from build123d import *

# Parameters (mm, degrees)
F1_DEPTH = 304.8


with BuildPart() as f1:
    # F0 (on Front) → F1 (new body)
    with BuildSketch(Plane.XZ):
        with BuildLine():
            Line((-9.986188, 0), (0, 0))
            Line((0, 0), (109.393812, 0))
            ThreePointArc((109.393812, 0), (110.663812, 0.340295), (111.593517, 1.27))
            Line((111.593517, 1.27), (-8.716188, 1.27))
            ThreePointArc((-8.716188, 1.27), (-10.512239, 2.013949), (-11.256188, 3.81))
            Line((-11.256188, 3.81), (-11.256188, 26.67))
            Line((-11.256188, 26.67), (-12.526188, 26.67))
            Line((-12.526188, 26.67), (-12.526188, 2.54))
            ThreePointArc((-12.526188, 2.54), (-11.782239, 0.743949), (-9.986188, 0))
        make_face()
    extrude(amount=-F1_DEPTH)


solid = f1.part
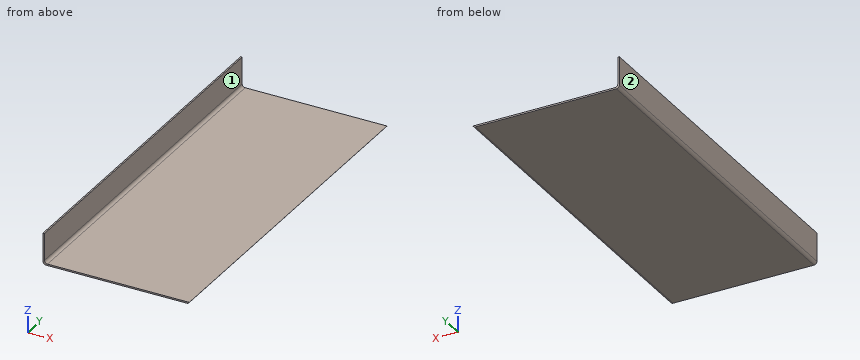
Could you check a few things on this model? Use its own coordinates, in mm. Face numbers are marked on the shaded views. A direction names the side the tool comes from. Give positions to 0.01 mm unless a question says otherwise; leave off trailing zeros. Write each loop counter-clockwise with the first axis right and the second up, starting at its lowest first coordinate (ties: lowest second). Pieces come first, ordered by that corner, then holes. Notation, with made-up numbers: (33.25, 65.25) -> (38.25, 65.25) arc R20 ccw to (38.25, 69.25) -> close; hole circle Ø7 at (-22, 0.25). An arc over 180 degrees is marked (long way). Answer as CSV lines item,"result". Start each with the question number.
(1) If we section it at C-C, the plane x = -2.5: Write out the boundary of the cut face in (y, z), and give its area (3 significant figures).
(2) I'm going to push a flat-ended pin straight in: pin 1 Ø4 at (y, z) = (247.5, 13) entering from +X. Where does the tip first touch, or does it pass through?
(3) If we section it at A-A, the plane y = 89: Write out the boundary of the cut face in (x, z).
(4) Which directions (+Z, -Z, +X, -X, +Y, -Y) give clear straight access to the entire face, cutting with the end or side of a thin tool? Please do the marked faces 1 and 2.
(5) If we section it at B-B, the plane z = 8.5: Write out the boundary of the cut face in (x, y), and give its area (3 significant figures).
(6) Please list where these lines run through material, in increasing order: line 1 (Z direction, x = 57.5, y = 255.5); line 2 (X direction, y = 74.5, z = 13.25); line 3 (X direction, y = 150.5, z = 3.5).
Answer list:
1,outline,"(0, 0) -> (304.8, 0) -> (304.8, 1.27) -> (0, 1.27) -> close"
1,area,"387 mm^2"
2,pin 1,"x = -11.26"
3,outline,"(-12.53, 2.54) arc R2.54 ccw to (-9.99, 0) -> (109.39, 0) arc R2.54 ccw to (111.59, 1.27) -> (-8.72, 1.27) arc R2.54 cw to (-11.26, 3.81) -> (-11.26, 26.67) -> (-12.53, 26.67) -> close"
4,face 1,"+Z, +X, +Y, -Y"
4,face 2,"+Z, -Z, -X, +Y, -Y"
5,outline,"(-12.53, 0) -> (-11.26, 0) -> (-11.26, 304.8) -> (-12.53, 304.8) -> close"
5,area,"387 mm^2"
6,line 1,"0 to 1.27"
6,line 2,"-12.53 to -11.26"
6,line 3,"-12.53 to -11.24"
